from build123d import *

# Parameters (mm, degrees)
SKETCH_1_W                 = 80
SKETCH_1_H                 = 80
EXTRUDE_278_DEPTH          = 21
EXTRUDE_2_DEPTH            = 21
HOLE_WIZARD_M6_D           = 6.6
HOLE_WIZARD_M6_CSINK_D     = 12.6
HOLE_WIZARD_M6_CSINK_ANGLE = 90
SKETCH_10_W                = 40
SKETCH_10_H                = 40
CUT_EXTRUDE_40_DEPTH       = 11.5
SKETCH_11_W                = 42.3
SKETCH_11_H                = 42.3
NEMA17_DEPTH               = 14
NEMA17_M3_D                = 3.4
NEMA17_M3_CSINK_D          = 6.3
NEMA17_M3_CSINK_ANGLE      = 90
FILLET_1_R                 = 2
SKETCH_14_R                = 15.5
NEMA23_DEPTH               = 106.588825166
SKETCH_2_W                 = 35
SKETCH_2_H                 = 88
CUT_EXTRUDE_4267_DEPTH     = 107.742681248
CUT_EXTRUDE_1_DEPTH        = 107.742681248
FILLET_2_R                 = 10
CHAMFER_1_SIZE             = 2.5


with BuildPart() as part:
    # Эскиз1 → Extrude 278 (new body)
    with BuildSketch(Plane(origin=(0, 0, 0), x_dir=(1, 0, 0), z_dir=(0, 1, 0))):
        Rectangle(SKETCH_1_W, SKETCH_1_H)
    extrude(amount=EXTRUDE_278_DEPTH)

    # Эскиз9 → База-2 (add)
    with BuildSketch(Plane(origin=(0, 21, 0), x_dir=(1, 0, 0), z_dir=(0, 1, 0))):
        Polygon((40, 40), (93, 40), (93, -48), (-40, -48), (-40, -40), (40, -40), align=None)
    extrude(amount=-EXTRUDE_2_DEPTH)

    # Крепление-M6 (through all)
    with Locations(Plane(origin=(0, 21, 0), x_dir=(1, 0, 0), z_dir=(0, 1, 0))):
        with Locations((-20, -20), (20, 20), (5.5, -5.5), (34.5, -5.5), (34.5, -34.5), (5.5, -34.5)):
            CounterSinkHole(HOLE_WIZARD_M6_D / 2, HOLE_WIZARD_M6_CSINK_D / 2, counter_sink_angle=HOLE_WIZARD_M6_CSINK_ANGLE)

    # Эскиз10 → Профиль-40 (cut)
    with BuildSketch(Plane.XZ):
        with Locations((20, 20)):
            Rectangle(SKETCH_10_W, SKETCH_10_H)
    extrude(amount=-CUT_EXTRUDE_40_DEPTH, mode=Mode.SUBTRACT)

    # Эскиз11 → Nema17 (cut)
    with BuildSketch(Plane.XZ):
        with Locations((65, 20)):
            Rectangle(SKETCH_11_W, SKETCH_11_H)
    extrude(amount=-NEMA17_DEPTH, mode=Mode.SUBTRACT)

    # Nema17-M3 (through all)
    with Locations(Plane(origin=(0, 21, 0), x_dir=(-1, 0, 0), z_dir=(0, 1, 0))):
        with Locations((-49.5, 35.5), (-80.5, 35.5), (-80.5, 4.5), (-49.5, 4.5)):
            CounterSinkHole(NEMA17_M3_D / 2, NEMA17_M3_CSINK_D / 2, counter_sink_angle=NEMA17_M3_CSINK_ANGLE)

    # Скругление1
    fillet_1_edges = [part.edges().sort_by_distance(p)[0] for p in [
        (0, 5.75, 0),
        (0, 5.75, 40),
        (40, 5.75, 40),
        (40, 5.75, 0),
        (86.15, 7, 41.15),
        (86.15, 7, -1.15),
        (43.85, 7, -1.15),
        (43.85, 7, 41.15),
    ]]
    fillet(fillet_1_edges, radius=FILLET_1_R)

    # Эскиз14 → Вырез-Nema23 (cut, through all)
    with BuildSketch(Plane.XZ.offset(-14)):
        with Locations(Location((65, 20, 0), (0, 0, 270))):
            Circle(SKETCH_14_R)
    extrude(amount=-NEMA23_DEPTH, mode=Mode.SUBTRACT)

    # Эскиз2 → Cut-Extrude 4267 (cut, through all)
    with BuildSketch(Plane(origin=(0, 21, 0), x_dir=(1, 0, 0), z_dir=(0, 1, 0))):
        with Locations((-22.5, -4)):
            Rectangle(SKETCH_2_W, SKETCH_2_H)
    extrude(amount=-CUT_EXTRUDE_4267_DEPTH, mode=Mode.SUBTRACT)

    # Эскиз15 → Вырез-Вытянуть1 (cut, through all)
    with BuildSketch(Plane(origin=(0, 21, 0), x_dir=(1, 0, 0), z_dir=(0, 1, 0))):
        Polygon((60, 40), (93, -4), (93, 40), align=None)
    extrude(amount=-CUT_EXTRUDE_1_DEPTH, mode=Mode.SUBTRACT)

    # Скругление2
    fillet_2_edges = [part.edges().sort_by_distance(p)[0] for p in [
        (93, 10.5, 48),
        (-5, 10.5, -40),
        (-5, 10.5, 48),
        (60, 10.5, -40),
        (93, 10.5, 4),
    ]]
    fillet(fillet_2_edges, radius=FILLET_2_R)

    # Фаска1
    chamfer_1_edges = [part.edges().sort_by_distance(p)[0] for p in [
        (65, 21, 35.5),
        (93, 21, 22.666666667),
        (77, 21, -17.333333333),
        (30, 21, -40),
        (-5, 21, 4),
        (44, 21, 48),
        (-2.071067812, 21, 45.071067812),
        (90.071067812, 21, 45.071067812),
        (-2.071067812, 21, -37.071067812),
        (59.472135955, 21, -38.94427191),
        (92.486832981, 21, 4.171055673),
    ]]
    chamfer(chamfer_1_edges, length=CHAMFER_1_SIZE)


solid = part.part
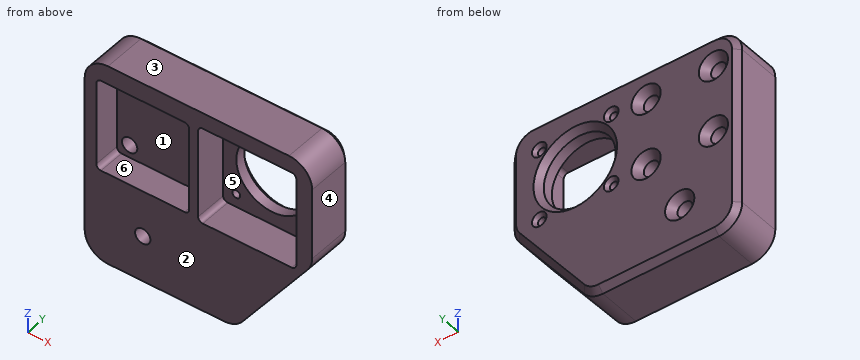
Verification items for the finished model (mm, model axes). Face numbers are marked on the shaded views. A direction names the side the tool comes from. Coordinates: 2 decimals unless noted, no trailing zeros. Order: outer loops, then holes, each group sorted by start corner. A loop starts at its lowest first (then second) coordinate and runs counter-clockwise, first axis right, second up.
Item 1: Release check for a two-part mould opening along X. For the marked faces 3, 4, 5 and 6 record: +X half, -X half, draft (parallel to the pull), parting line (faces both ways), or undercut.
Filled in:
face 3: draft
face 4: +X half
face 5: undercut
face 6: undercut
Item 2: Depth check by flat-ended pin: pin 1 (5.5 mm diameter, centred on x = 80.5, z = 4.5, fed in from +Y); pin 2 (12 mm diameter, centred on y = 8, z = -5, fed in from +X); pin 3 (2 mm diameter, centred on x = 27, z = 31, fed in from -Y). Enter the tip coordinate at first touch or a pass-through.
Filled in:
pin 1: stops at y = 20.6
pin 2: stops at x = 90.75
pin 3: stops at y = 11.5
Item 3: Section check A-A, the plane x = 20. Enter the section's corners in (y, z).
Filled in:
outline: (0, -40) - (18.5, -40) - (21, -37.5) - (21, -26.3) - (18, -23.3) - (0, -23.3) - close; (0, -16.7) - (18, -16.7) - (21, -13.7) - (21, 45.5) - (18.5, 48) - (0, 48) - (0, 40) - (11.5, 40) - (11.5, 0) - (0, 0) - close
Item 4: Section check B-B, the plane y = 7. Enter the section's corners in (x, z), then the cut area to 3 significant figures.
Filled in:
outline: (-5, -30) arc R10 ccw to (5, -40) - (55, -40) arc R10 ccw to (63, -36) - (91, 1.33) arc R10 ccw to (93, 7.33) - (93, 38) arc R10 ccw to (83, 48) - (5, 48) arc R10 ccw to (-5, 38) - close; hole (0, 2) arc R2 ccw to (2, 0) - (38, 0) arc R2 ccw to (40, 2) - (40, 38) arc R2 ccw to (38, 40) - (2, 40) arc R2 ccw to (0, 38) - close; hole circle Ø6.6 at (20, -20); hole (43.85, 0.85) arc R2 ccw to (45.85, -1.15) - (84.15, -1.15) arc R2 ccw to (86.15, 0.85) - (86.15, 39.15) arc R2 ccw to (84.15, 41.15) - (45.85, 41.15) arc R2 ccw to (43.85, 39.15) - close
area: 4,410 mm2
Item 5: Material ranges on L1, parallel to X at y = 2.5, z = 9; L2, parallel to Z at x = 34.5, y = 14.5; L3, parallel to Z at x = 46, y = 2.25, recorded low to high.
Filled in:
L1: x = -5 to 0, 40 to 43.85, 86.15 to 93
L2: z = -40 to 2.2, 8.8 to 31.2, 37.8 to 48
L3: z = -40 to -1.15, 41.15 to 48
Item 6: Section check C-C, the plane x = 34.5. Enter the section's corners in (y, z).
Filled in:
outline: (0, -40) - (18.5, -40) - (21, -37.5) - (21, -0.8) - (18, 2.2) - (11.5, 2.2) - (11.5, 0) - (0, 0) - close; (0, 40) - (11.5, 40) - (11.5, 37.8) - (18, 37.8) - (21, 40.8) - (21, 45.5) - (18.5, 48) - (0, 48) - close; (11.5, 8.8) - (18, 8.8) - (21, 11.8) - (21, 28.2) - (18, 31.2) - (11.5, 31.2) - close
Item 7: Access from +Z, -Z, +X, -X, +Y, -Y to the whole of each face (thin tool, end or side, straight path). Record for the marked faces 1 and 2.
Filled in:
face 1: -Y
face 2: +Z, -Z, +X, -X, -Y
Item 8: Section check D-D, the plane y = 12.75. Enter the section's corners in (x, z), then the cut area to 3 significant figures.
Filled in:
outline: (-5, -30) arc R10 ccw to (5, -40) - (55, -40) arc R10 ccw to (63, -36) - (91, 1.33) arc R10 ccw to (93, 7.33) - (93, 38) arc R10 ccw to (83, 48) - (5, 48) arc R10 ccw to (-5, 38) - close; hole circle Ø6.6 at (5.5, 5.5); hole circle Ø6.6 at (5.5, 34.5); hole circle Ø6.6 at (20, -20); hole circle Ø6.6 at (34.5, 5.5); hole circle Ø6.6 at (34.5, 34.5); hole (43.85, 0.85) arc R2 ccw to (45.85, -1.15) - (84.15, -1.15) arc R2 ccw to (86.15, 0.85) - (86.15, 39.15) arc R2 ccw to (84.15, 41.15) - (45.85, 41.15) arc R2 ccw to (43.85, 39.15) - close
area: 5,870 mm2
